Part model, mm, in its own coordinate system. A direction names the side the tool comes from. Round coordinates to 2 decimals unless told otherwise and drop trailing zeros. Write each loop counter-clockwise with the first axis right and the second up, starting at its lowest first coordinate (ties: lowest second). Pieces come first, ordered by that corner, then holes.
from build123d import *

# Parameters (mm, degrees)
SKETCH_1_R          = 14.1
EXTRUDE_1_DEPTH     = 94
SKETCH_2_R          = 12.5
CUT_EXTRUDE_1_DEPTH = 92
FILLET_2_R          = 1
FILLET_3_R          = 1
FILLET_4_R          = 1
SKETCH_3_R          = 8
CUT_EXTRUDE_2_DEPTH = 2


with BuildPart() as part:
    # Эскиз1 → Бобышка-Вытянуть1 (new body)
    with BuildSketch(Plane(origin=(0, 0, 0), x_dir=(1, 0, 0), z_dir=(0, 1, 0))):
        with Locations(Location((0, 0, 0), (0, 0, 270))):
            Circle(SKETCH_1_R)
    extrude(amount=EXTRUDE_1_DEPTH)

    # Эскиз2 → Вырез-Вытянуть1 (cut)
    with BuildSketch(Plane.XZ):
        with Locations(Location((0, 0, 0), (0, 0, 270))):
            Circle(SKETCH_2_R)
    extrude(amount=-CUT_EXTRUDE_1_DEPTH, mode=Mode.SUBTRACT)

    # Скругление2
    fillet_2_edges = [part.edges().sort_by_distance(p)[0] for p in [
        (0, 0, 12.5),
    ]]
    fillet(fillet_2_edges, radius=FILLET_2_R)

    # Скругление3
    # the kernel refuses this fillet: 1 mm, written as the material it takes off along each edge
    with BuildSketch(Plane(origin=(0, 0, 0), x_dir=(0, 0, 1), z_dir=(-1, 0, 0))) as fillet_3_piece_1:
        with BuildLine():
            CenterArc((13.1, 0.916515139), FILLET_3_R, 293.578178478, 66.421821522)
            Line((14.1, 0.916515139), (14.12, 0.916515139))
            Line((14.12, 0.916515139), (14.12, 0))
            Line((14.12, 0), (14.1, -0.02))
            ThreePointArc((14.1, -0.02), (13.8, -0.02), (13.508, -0.018330303))
            Line((13.508, -0.018330303), (13.5, 0))
        make_face()
    revolve(axis=Axis((0, 0, 0), (0, 1, 0)), mode=Mode.SUBTRACT)

    # Скругление4
    fillet_4_edges = [part.edges().sort_by_distance(p)[0] for p in [
        (0, 94, -14.1),
    ]]
    fillet(fillet_4_edges, radius=FILLET_4_R)

    # Эскиз3 → Вырез-Вытянуть2 (cut)
    with BuildSketch(Plane(origin=(0, 94, 0), x_dir=(1, 0, 0), z_dir=(0, 1, 0))):
        with Locations(Location((0, 0, 0), (0, 0, 270))):
            Circle(SKETCH_3_R)
    extrude(amount=-CUT_EXTRUDE_2_DEPTH, mode=Mode.SUBTRACT)


solid = part.part
Q1. Saw through at A-A, the plane z = 0. Write the cut outline in (x, y).
Q2. Tool access for faces 4 (the cylindrical face through (-7.81, 93.01, -1.73)), 5 (the flat face through (-8.2, 92, 0.2)): list every direction of +Z, -Z, +X, -X, +Y, -Y with a clear straight run to the whole face (end or side of a thin tool).
Q3. Drop flat-ended pins along their axis: P1, Ø2, axis at y = 44.5, z = -9.5, coming from the +X side; P2, Ø8, axis at x = -2.5, z = -9, coming from the -Y side; P3, Ø4, axis at x = -6.5, z = -8.5, coming from the -Y side. Give the stop position or say it passes through.
Q4. Wall check: line 1 (X direction, y = 92.6, z = 0); line 2 (Z direction, x = 0.5, y = 5); line 3 (Y direction, x = -9, z = 8). Give the ranges that are in metal, low to high.
Q5. Saw through at B-B, the plane y = 71. Write the cut outline in (x, z).
Q6. Two-plate mould, pull along X, no slides. Class faces 1 (the cylindrical face through (-5.4, 46.314, 13.025)), 2 (the flat face through (-6, 94, -6)), 3 (the cylindrical face through (3.755, 45.863, -11.923)): released by +X, released by -X, zero draft, split by the parting line, or undercut.
Computed:
1. outline: (-14.1, 0.92) arc R1 ccw to (-13.5, 0) arc R1 ccw to (-12.5, 1) - (-12.5, 92) - (-8, 92) - (-8, 94) - (-13.1, 94) arc R1 ccw to (-14.1, 93) - close; (8, 92) - (12.5, 92) - (12.5, 1) arc R1 ccw to (13.5, 0) arc R1 ccw to (14.1, 0.92) - (14.1, 93) arc R1 ccw to (13.1, 94) - (8, 94) - close
2. face 4: +Y, -Y
2. face 5: -Y
3. P1: stops at x = 11.25
3. P2: stops at y = 0.01
3. P3: stops at y = 0.4
4. line 1: x = -14.1 to -8, 8 to 14.1
4. line 2: z = -14.09 to -12.49, 12.49 to 14.09
4. line 3: y = 92 to 94
5. outline: circle Ø28.2 at (0, 0); hole circle Ø25 at (0, 0)
6. face 1: split by the parting line
6. face 2: zero draft
6. face 3: undercut
